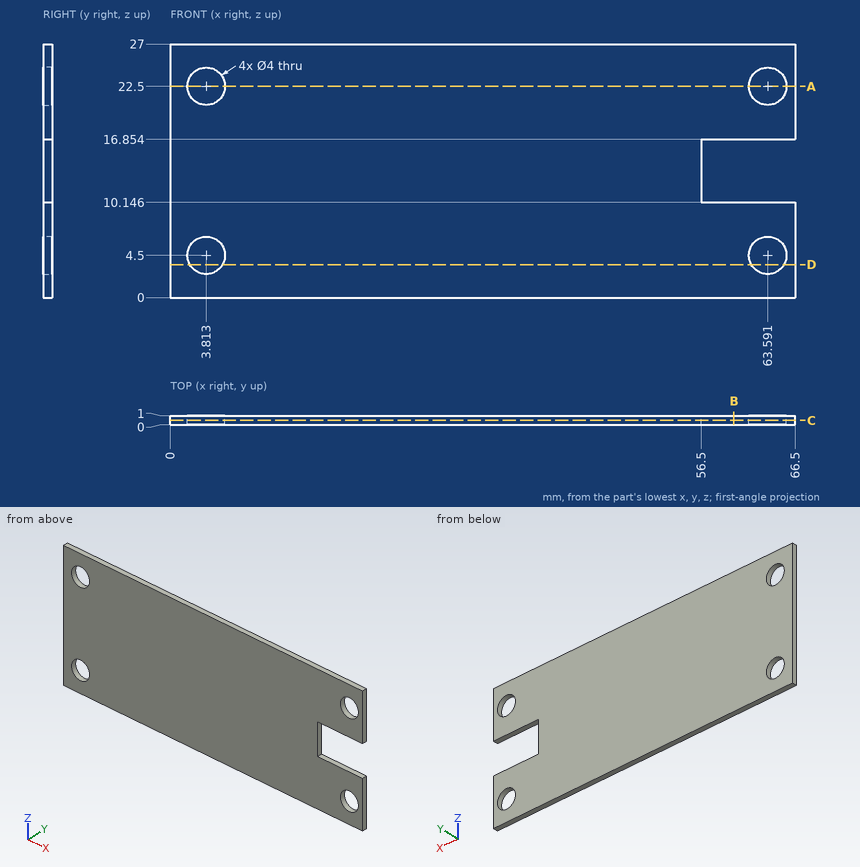
Answer from the drawing. Dimensions are ordinates in mm from the lowest x, y and z of the part. Round coordinates to 2 decimals unless told otherwise and drop trailing zeros. Order: outer loops, then holes, each group sorted by start corner. A loop starts at its lowest first (then second) coordinate and runs counter-clockwise, first axis right, second up. Notation, with made-up numbers: (78, 23.5) -> (89, 23.5) arc R20 ccw to (89, 44.5) -> close; hole circle Ø9 at (19.25, 8.5). An arc over 180 degrees is marked (long way). Answer as CSV lines item,"result".
Q1. A cutting plane is placed at D-D on z = 3.5. Determine the outline of the cut face in (x, y) (1 decimal).
Computed values:
outline,"(0, 0) -> (2.1, 0) -> (2.1, 1) -> (0, 1) -> close; (5.5, 0) -> (61.9, 0) -> (61.9, 1) -> (5.5, 1) -> close; (65.3, 0) -> (66.5, 0) -> (66.5, 1) -> (65.3, 1) -> close"
Q2. A cutting plane is placed at A-A on z = 22.5. Determine the outline of the cut face in (x, y).
Computed values:
outline,"(0, 0) -> (1.81, 0) -> (1.81, 1) -> (0, 1) -> close; (5.81, 0) -> (61.59, 0) -> (61.59, 1) -> (5.81, 1) -> close; (65.59, 0) -> (66.5, 0) -> (66.5, 1) -> (65.59, 1) -> close"
Q3. A cutting plane is placed at C-C on y = 0.5. Determine the outline of the cut face in (x, z).
Computed values:
outline,"(0, 0) -> (66.5, 0) -> (66.5, 10.15) -> (56.5, 10.15) -> (56.5, 16.85) -> (66.5, 16.85) -> (66.5, 27) -> (0, 27) -> close; hole circle Ø4 at (3.81, 4.5); hole circle Ø4 at (3.81, 22.5); hole circle Ø4 at (63.59, 4.5); hole circle Ø4 at (63.59, 22.5)"
Q4. Given pin 1 (3 mm diameter, centred on x = 63.59, z = 4.5, fed in from -Y), flat-ended and moving along its own axis, determine where the tip first touches the part or whether it passes through.
Computed values:
pin 1,"passes through"
Q5. A cutting plane is placed at B-B on x = 60. Determine the outline of the cut face in (y, z), plus the area to 3 significant figures.
Computed values:
outline,"(0, 0) -> (1, 0) -> (1, 10.15) -> (0, 10.15) -> close; (0, 16.85) -> (1, 16.85) -> (1, 27) -> (0, 27) -> close"
area,"20.3 mm^2"
Q6. Consider line 1 (Z direction, x = 59, y = 0.75); line 2 (X direction, y = 0.4, z = 22.5); line 3 (X direction, y = 0.75, z = 12.75). Determine where each line is inside the solid, lowest interval first. Write a range as from..to.
Computed values:
line 1,"z = 0..10.15, 16.85..27"
line 2,"x = 0..1.81, 5.81..61.59, 65.59..66.5"
line 3,"x = 0..56.5"
